```python
from build123d import *

# Parameters (mm, degrees)
F0_R     = 16.9
F1_DEPTH = 23


with BuildPart() as f1:
    # F0 (on Top) → F1 (new body)
    with BuildSketch(Plane.XY):
        Circle(F0_R)
        Polygon((-9.5, -1.65), (-9.5, 0), (-9.5, 1.65), (0, 1.65), (9.5, 1.65), (9.5, 0), (9.5, -1.65), (0, -1.65), align=None, mode=Mode.SUBTRACT)
    extrude(amount=F1_DEPTH)


solid = f1.part
```
Geometry: final body of the model. Coordinates: model frame, mm. A direction names the side the tool comes from. Give positions to 0.01 mm unless a question says otherwise; leave off trailing zeros. Write each loop counter-clockwise with the first axis right and the second up, starting at its lowest first coordinate (ties: lowest second). Pieces come first, ordered by that corner, then holes.
1. Pin query (flat end, axial travel): P1, Ø6, axis at y = 5.5, z = 14, coming from the -X side; P2, Ø6, axis at y = -4.5, z = 10, coming from the -X side; P3, Ø6, axis at y = -11.5, z = 17.5, coming from the -X side. Return the tip coordinate at first contact, or that it passes through.
2. Section query B-B, the plane y = 0. Return loops of the section in (x, z), then the cut area to 3 significant figures.
3. Section query A-A, the plane x = 0. Return loops of the section in (y, z), then the cut area to 4 significant figures.
4. Reachability of faces 1 (the flat face through (0, -4, 23)), 2 (the flat face through (9.5, 0, 11)) from +Z, -Z, +X, -X, +Y, -Y: full face, straight path, thin tool, end or side. Return the list, or none.
5. Section query D-D, the plane y = 12. Return loops of the section in (x, z), then the cut area to 3 significant figures.
6. Draft query along Y for faces 3 (the flat face through (0, -4, 0)), 4 (the cylindrical face through (16.12, 5.08, 11.34)), 5 (the flat face through (0, 1.65, 11)), 6 (the flat face through (-9.5, 0, 11)). Return one class per face: released by +Y, released by -Y, zero draft, split by the parting line, or undercut.
7. Section query C-C, the plane z = 8.75. Return loops of the section in (x, y).
8. Line query: probe 1 along Y at (x, z) = (-2, 12.75); probe 2 along Y at (x, z) = (8.5, 13.5); probe 3 along X at (y, z) = (-10.5, 11). Output: solid intervals per line, ascending.
Computed:
1. P1: stops at x = -16.71
1. P2: stops at x = -16.83
1. P3: stops at x = -14.61
2. outline: (-16.9, 0) - (-9.5, 0) - (-9.5, 23) - (-16.9, 23) - close; (9.5, 0) - (16.9, 0) - (16.9, 23) - (9.5, 23) - close
2. area: 340 mm2
3. outline: (-16.9, 0) - (-1.65, 0) - (-1.65, 23) - (-16.9, 23) - close; (1.65, 0) - (16.9, 0) - (16.9, 23) - (1.65, 23) - close
3. area: 701.5 mm2
4. face 1: +Z, +X, -X, +Y, -Y
4. face 2: +Z, -Z
5. outline: (-11.9, 0) - (11.9, 0) - (11.9, 23) - (-11.9, 23) - close
5. area: 547 mm2
6. face 3: zero draft
6. face 4: split by the parting line
6. face 5: undercut
6. face 6: undercut
7. outline: circle Ø33.8 at (0, 0); hole (-9.5, -1.65) - (9.5, -1.65) - (9.5, 1.65) - (-9.5, 1.65) - close
8. probe 1: y = -16.78 to -1.65, 1.65 to 16.78
8. probe 2: y = -14.61 to -1.65, 1.65 to 14.61
8. probe 3: x = -13.24 to 13.24
